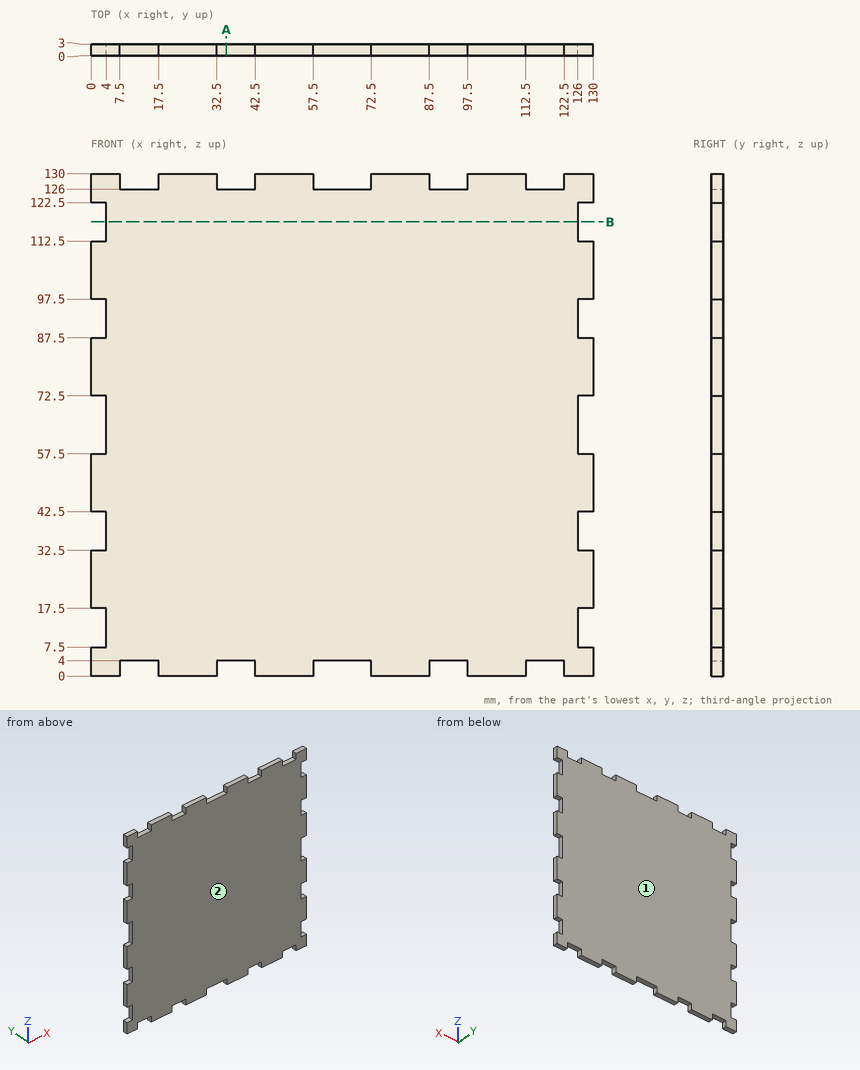
Geometry check sheet. Reference: drawing and pictorial views, mm from the part's lowest x, y, z. Give positions to 0.01 mm unless a question says otherwise; leave off trailing zeros. Write each loop counter-clockwise with the first axis right and the second up, starting at its lowest first coordinate (ties: lowest second). Pieces come first, ordered by that corner, then holes. Notation, with made-up numbers: M -13.5,-12.5 L 31.5,-12.5 A22 cw 31.5,-0.5 Z; hole C 63.5,-38 d1. An arc over 180 degrees is marked long. Put each result on its own line as item: value. Start each with the question number.
1. Scan line: line 1 along Z through (x, y) = (90, 2.55). Record every from-to range of solid material in increasing order. Write a range as [from, to].
2. Draft check along Y on the marked faces 1 and 2. Enter one of: +Y half, -Y half, draft (parallel to the pull), parting line (faces both ways), or undercut.
3. Go/stop test with a flat-tipped pin: pin 1 Ø1.5 at (y, z) = (1.5, 116.5) entering from +X. Record where the tip stops, or that it passes through.
4. Section check A-A (x = 35). Record the cut outline in (y, z).
5. Section check B-B (z = 117.5). Record the cut outline in (x, y), and give its area (3 significant figures).
Answer list:
1. line 1: [4, 126]
2. face 1: +Y half
2. face 2: -Y half
3. pin 1: x = 126
4. outline: M 0,4 L 3,4 L 3,126 L 0,126 Z
5. outline: M 4,0 L 126,0 L 126,3 L 4,3 Z
5. area: 366 mm2
